Can you work these out from the model? Positions are in its coordinate system, mm. Face numbers are marked on the shaded views. A direction names the side the tool comes from. Give positions to 0.01 mm unless a question says otherwise; leave off trailing zeros. Order: outer loops, then holes, each group sorted by start corner. A loop starts at its lowest first (then second) coordinate and runs counter-clockwise, first axis right, second up. Notation, with made-up numbers: (51.5, -3.75) -> (56.5, -3.75) arc R13 ccw to (56.5, 3.25) -> close; hole circle Ø10 at (63.25, -9.75). An arc over 180 degrees is marked (long way). Answer as a JSON object with one key per item and string values.
Autodesk Inventor part; units mm, degrees
ref_plane "Work Plane1" through (0, 10, 5.1) normal (0, -1, 0) x (1, 0, 0)
ref_plane "YZ Plane" through (0, 0, 0) normal (1, 0, 0) x (0, 1, 0)
ref_plane "XZ Plane" through (0, 0, 0) normal (0, 1, 0) x (-1, 0, 0)
sketch "Sketch1" plane through (0, 0, 0) normal (1, 0, 0) x (0, 1, 0)
  arc A0 (0, -5.1) -> (0, 5.1) centre (0, 0) ccw
  arc A1 (0, -10) -> (0, 10) centre (0, 0) ccw
  line L0 (0, 10) -> (0, 5.1)
  line L1 (0, -5.1) -> (0, -10)
  dimension "d0" = 10.2
  dimension "d1" = 20
extrude "Extrusion1" add sketch "Sketch1" along normal blind 9.8
sketch "Sketch2" plane through (0, 0, 5.1) normal (0, -1, 0) x (1, 0, 0)
  line L0 (0, 4.9) -> (0, 0)
  line L1 (0, 0) -> (9.8, 0)
  line L2 (0, 4.9) -> (9.8, 0)
  line L3 (0, -10.2) -> (9.8, -10.2)
  line L4 (0, -15.1) -> (9.8, -15.1)
  line L5 (0, -10.2) -> (9.8, -15.1)
  point P0 (0, -5.1)
  point P1 (4.9, 2.45)
  point P2 (4.9, -12.65)
hole "Hole1" at (4.9, 0, 7.55) at (4.9, 0, -7.55) direction (0, 1, 0) diameter 3 end through all countersink diameter 3.5 countersink angle 90
ref_plane "Work Plane1" through (0, 10, 5.1) normal (0, -1, 0) x (1, 0, 0)
sketch "Sketch3" plane through (0, 10, 5.1) normal (0, -1, 0) x (1, 0, 0)
  circle A0 centre (4.9, -12.65) radius 1.5
  circle A1 centre (4.9, -12.65) radius 3
  circle A2 centre (4.9, 2.45) radius 1.5
  circle A3 centre (4.9, 2.45) radius 3
  point P0 (0, -5.1)
  dimension "d12" = 6
  dimension "d13" = 6
extrude "Extrusion2" cut sketch "Sketch3" along normal blind 6 contours A0 | A1 | A2 | A3
chamfer "Chamfer1" distance 2 angle 45 2 edges at (9.8, 5.1, 0) (0, 5.1, 0)
chamfer "Chamfer2" distance 0.5 angle 45 14 edges at (9.8, 10, 0) (9.8, 0, 8.55) (4.9, 0, 10) (0, 10, 0) (9.8, 0, -8.55) (8.8, 0, -6.1) (4.9, 0, -5.1) (0, 0, 8.55) (1, 0, 6.1) (4.9, 0, 5.1) (8.8, 0, 6.1) (1, 0, -6.1) (0, 0, -8.55) (4.9, 0, -10)
properties part number "ForkTop"
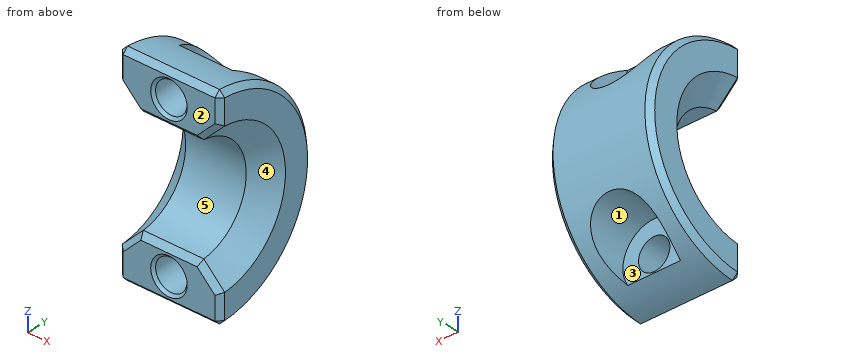
1. Will these pins go through, and if not, where does the flat tip stop? pin 1 Ø1.8 at (x, z) = (4.9, 7.55) entering from -Y; pin 2 Ø1.4 at (x, z) = (3.5, -7.5) entering from +Y; pin 3 Ø5 at (x, z) = (5.5, -4) entering from +Y; pin 4 Ø1.5 at (x, z) = (6, 3) entering from -Y.
Worked answers:
{"pin 1": "through", "pin 2": "y = 4", "pin 3": "y = 9.89", "pin 4": "y = 3.46"}
2. For the marked faces 1 and 2, which set-ups out of +Z, -Z, +X, -X, +Y, -Y let a thin tool reach every point of the face, with its end or its side?
Worked answers:
{"face 1": "+Y", "face 2": "+Z, -Z, +X, -X, -Y"}
3. If we section it at A-A on x = 4.9: Please give me the cut outline in (y, z).
Worked answers:
{"outline": "(0, -9.5) -> (0.5, -9.99) arc R10 ccw to (4, -9.17) -> (4, -9.05) -> (0.25, -9.05) -> (0, -9.3) -> close; (0, -5.8) -> (0.25, -6.05) -> (4, -6.05) -> (4, -4.55) -> (8.9, -4.55) arc R10 ccw to (8.9, 4.55) -> (4, 4.55) -> (4, 6.05) -> (0.25, 6.05) -> (0, 5.8) -> (0, 5.6) -> (0.5, 5.08) arc R5.1 cw to (0.5, -5.08) -> (0, -5.6) -> close; (0, 9.3) -> (0.25, 9.05) -> (4, 9.05) -> (4, 9.17) arc R10 ccw to (0.5, 9.99) -> (0, 9.5) -> close"}
4. If we mould it in two halves opening along X, with no side actions, what happens to the marked faces 3, 4 and 5? For each: +X half, -X half, draft (parallel to the pull), parting line (faces both ways), or undercut.
Worked answers:
{"face 3": "undercut", "face 4": "+X half", "face 5": "draft"}
5. Please list where these lines run through material, in increasing order: L1, parallel to Z at x = 4, y = 1.5; L2, parallel to Z at x = 4.9, y = 2.8; L3, parallel to Z at x = 4.9, y = 6.45.
Worked answers:
{"L1": "-9.89 to -8.75, -6.35 to -4.87, 4.87 to 6.35, 8.75 to 9.89", "L2": "-9.6 to -9.05, -6.05 to -4.26, 4.26 to 6.05, 9.05 to 9.6", "L3": "-4.55 to 4.55"}
